Build history of the part. All positions in model axes, mm. Round coordinates to 2 decimals unless told otherwise and drop trailing zeros. Loops run counter-clockwise (first coordinate to the right, second up) from the corner with the lowest first, then second, coordinate; pieces in that order, holes last. Notation, with made-up numbers: M -13,69.25 L 20,69.25 A20 cw 20,102.25 Z; hole C 38.25,37.5 d4. An arc over 180 degrees is marked long. Write each question's results on one line, items separated by ' | '. Start each with the question number.
```python
from build123d import *

# Parameters (mm, degrees)
SKETCH1_W           = 75
SKETCH1_H           = 55
BOSS_EXTRUDE1_DEPTH = 3


with BuildPart() as part:
    # Sketch1 → Boss-Extrude1 (new body)
    with BuildSketch(Plane(origin=(0, 0, 0), x_dir=(0, 1, 0), z_dir=(0, 0, 1))):
        Rectangle(SKETCH1_W, SKETCH1_H)
    extrude(amount=BOSS_EXTRUDE1_DEPTH)

    # Cut-Extrude1 cone 1 section (through the dimple's axis) → Cut-Extrude1 (revolve, cut)
    with BuildSketch(Plane(origin=(-23.5, 33.5, 3), x_dir=(0, -1, 0), z_dir=(1, 0, 0))):
        Polygon((0, 0), (1.6, 0), (0, 18.288083684), align=None)
    revolve(axis=Axis((-23.5, 33.5, 3), (0, 0, -1)), mode=Mode.SUBTRACT)

    # Cut-Extrude1 cone 2 section (through the dimple's axis) → Cut-Extrude1 cone 2 (revolve, cut)
    with BuildSketch(Plane(origin=(23.5, 33.5, 3), x_dir=(0, -1, 0), z_dir=(1, 0, 0))):
        Polygon((0, 0), (1.6, 0), (0, 18.288083684), align=None)
    revolve(axis=Axis((23.5, 33.5, 3), (0, 0, -1)), mode=Mode.SUBTRACT)

    # Cut-Extrude1 cone 3 section (through the dimple's axis) → Cut-Extrude1 cone 3 (revolve, cut)
    with BuildSketch(Plane(origin=(-23.5, -33.5, 3), x_dir=(0, -1, 0), z_dir=(1, 0, 0))):
        Polygon((0, 0), (1.6, 0), (0, 18.288083684), align=None)
    revolve(axis=Axis((-23.5, -33.5, 3), (0, 0, -1)), mode=Mode.SUBTRACT)

    # Cut-Extrude1 cone 4 section (through the dimple's axis) → Cut-Extrude1 cone 4 (revolve, cut)
    with BuildSketch(Plane(origin=(23.5, -33.5, 3), x_dir=(0, -1, 0), z_dir=(1, 0, 0))):
        Polygon((0, 0), (1.6, 0), (0, 18.288083684), align=None)
    revolve(axis=Axis((23.5, -33.5, 3), (0, 0, -1)), mode=Mode.SUBTRACT)


solid = part.part
```
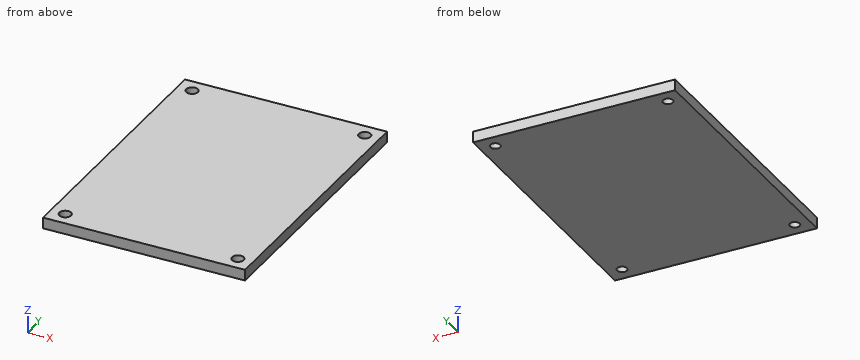
Item 1: Drill centre line: line 1 along Y through (x, z) = (24, 2.1). Where is it in solid material? Low to high. Write a range as [from, to].
Item 2: Saw through at B-B, the plane y = 33.5. Give the cut face in (x, z), then the cut area to 3 significant figures.
Item 3: Saw through at A-A, the plane x = -23.5. Give the cut face in (y, z), then the cut area to 3 significant figures.
Working result:
1) line 1: y = [-37.5, -34.94], [-32.06, 32.06], [34.94, 37.5]
2) outline: M -27.5,0 L -24.84,0 L -25.1,3 L -27.5,3 Z; M -22.16,0 L 22.16,0 L 21.9,3 L -21.9,3 Z; M 24.84,0 L 27.5,0 L 27.5,3 L 25.1,3 Z | area: 147 mm²
3) outline: M -37.5,0 L -34.84,0 L -35.1,3 L -37.5,3 Z; M -32.16,0 L 32.16,0 L 31.9,3 L -31.9,3 Z; M 34.84,0 L 37.5,0 L 37.5,3 L 35.1,3 Z | area: 207 mm²
